from build123d import *

# Parameters (mm, degrees)
F0_W           = 88.9
F0_H           = 63.5
F1_DEPTH       = 6.35
F2_D           = 8.2042
F3_D           = 3.3
F3_CBORE_D     = 8.25
F3_CBORE_DEPTH = 4


# Not quite as in the source:
# - a feature names something its author has since deleted; it is built from what else it names


with BuildPart() as f1:
    # F0 (on Top) → F1 (new body)
    with BuildSketch(Plane.XY):
        Rectangle(F0_W, F0_H)
    extrude(amount=F1_DEPTH)

    # F2 (through all)
    with Locations(Plane(origin=(0, 0, 0), x_dir=(1, 0, 0), z_dir=(0, 0, -1))):
        with Locations((-34.45, 21.75), (34.45, 21.75)):
            Hole(F2_D / 2)

    # F3 (through all)
    with Locations(Plane(origin=(0, 0, 0), x_dir=(1, 0, 0), z_dir=(0, 0, -1))):
        with Locations((-19.05, -19.05), (-19.05, 4.95), (20.95, -19.05), (20.95, 4.95)):
            CounterBoreHole(F3_D / 2, F3_CBORE_D / 2, F3_CBORE_DEPTH)


solid = f1.part
The listing builds one solid part. Answer for the finished solid, in the listing's coordinates (mm). A direction names the side the tool comes from. Coordinates: 2 decimals unless noted, no trailing zeros. Loops run counter-clockwise (first coordinate to the right, second up) from the corner with the lowest first, then second, coordinate; pieces in that order, holes last. Notation, with made-up numbers: (36.25, -11) -> (43.25, -11) arc R25 cw to (43.25, 24) -> close; hole circle Ø8 at (10, 36.25). An arc over 180 degrees is marked (long way). Answer in a Markdown table with one row per item. Add a question column.
1. The part is cut by section D-D, the plane z = 2. Write down the section's boundary in (x, y) (3 decimals).
2. The part is cut by section C-C, the plane x = 20.95. Write down the section's boundary in (y, z) (3 decimals), then the cut area to 3 significant figures.
3. Determine the mould class of faces 1 (the flat face through (-44.45, 0, 3)), 2 (the flat face through (-1, 31.75, 3)), 3 (the flat face through (44.45, 0, 3)), 4 (the flat face through (-19, -3, 4)) for opening direction X: +X half, -X half, draft (parallel to the pull), parting line (faces both ways), or undercut.
4. For faces 5 (the flat face through (21, 21, 4)), 6 (the flat face through (-1, 0, 6.35)), determine the directions among +Z, -Z, +X, -X, +Y, -Y from which every point of the face is accessible in a straight line to the end or side of a thin tool.
5. Consider line 1 (Y direction, x = 21, z = 6.25); line 2 (X direction, y = 19.05, z = 2.2) (3 decimals); line 3 (Y direction, x = -19.05, z = 1.2) (3 decimals). Determine where each line is inside the solid, lowest interval first. Write a range as [from, to].
6. The part is cut by section A-A, the plane x = -34.45. Write down the section's boundary in (y, z), then the cut area to 3 significant figures.
7. A flat-ended cylindrical pin translates along its axis: P1, Ø4, axis at x = -19.05, y = -4.95, coming from the -Z side. Find the tip coordinate at first contact, or state that the pin passes through.
8. The part is cut by section B-B, the plane y = 19.05. Write down the section's boundary in (x, z) (3 decimals), then the cut area to 3 significant figures.
Answer below:
| question | item | result |
|---|---|---|
| 1 | outline | (-44.45, -31.75) -> (44.45, -31.75) -> (44.45, 31.75) -> (-44.45, 31.75) -> close; hole circle Ø8.204 at (-34.45, -21.75); hole circle Ø8.25 at (-19.05, -4.95); hole circle Ø8.25 at (-19.05, 19.05); hole circle Ø8.25 at (20.95, -4.95); hole circle Ø8.25 at (20.95, 19.05); hole circle Ø8.204 at (34.45, -21.75) |
| 2 | outline | (-31.75, 0) -> (-9.075, 0) -> (-9.075, 4) -> (-6.6, 4) -> (-6.6, 6.35) -> (-31.75, 6.35) -> close; (-3.3, 4) -> (-0.825, 4) -> (-0.825, 0) -> (14.925, 0) -> (14.925, 4) -> (17.4, 4) -> (17.4, 6.35) -> (-3.3, 6.35) -> close; (20.7, 4) -> (23.175, 4) -> (23.175, 0) -> (31.75, 0) -> (31.75, 6.35) -> (20.7, 6.35) -> close |
| 2 | area | 322 mm2 |
| 3 | face 1 | -X half |
| 3 | face 2 | draft |
| 3 | face 3 | +X half |
| 3 | face 4 | undercut |
| 4 | face 5 | -Z |
| 4 | face 6 | +Z, +X, -X, +Y, -Y |
| 5 | line 1 | [-31.75, -6.6], [-3.3, 17.4], [20.7, 31.75] |
| 5 | line 2 | [-44.45, -23.175], [-14.925, 16.825], [25.075, 44.45] |
| 5 | line 3 | [-31.75, -9.075], [-0.825, 14.925], [23.175, 31.75] |
| 6 | outline | (-31.75, 0) -> (-25.85, 0) -> (-25.85, 6.35) -> (-31.75, 6.35) -> close; (-17.65, 0) -> (31.75, 0) -> (31.75, 6.35) -> (-17.65, 6.35) -> close |
| 6 | area | 351 mm2 |
| 7 | P1 | z = 4 |
| 8 | outline | (-44.45, 0) -> (-23.175, 0) -> (-23.175, 4) -> (-20.7, 4) -> (-20.7, 6.35) -> (-44.45, 6.35) -> close; (-17.4, 4) -> (-14.925, 4) -> (-14.925, 0) -> (16.825, 0) -> (16.825, 4) -> (19.3, 4) -> (19.3, 6.35) -> (-17.4, 6.35) -> close; (22.6, 4) -> (25.075, 4) -> (25.075, 0) -> (44.45, 0) -> (44.45, 6.35) -> (22.6, 6.35) -> close |
| 8 | area | 483 mm2 |
